Source: three-view drawing plus pictorial views. Frame: mm from the lowest corner of the part. A direction names the side the tool comes from. Round coordinates to 2 decimals unless told otherwise and drop trailing zeros. Order: outer loops, then holes, each group sorted by start corner. A loop starts at its lowest first (then second) coordinate and runs counter-clockwise, first axis right, second up. Notation, with made-up numbers: (4.25, -32) -> (58.25, -32) arc R24 cw to (58.25, 7) -> close; hole circle Ø9 at (-14, -23.5). An arc over 180 degrees is marked (long way). Use a Markdown table: item, result.
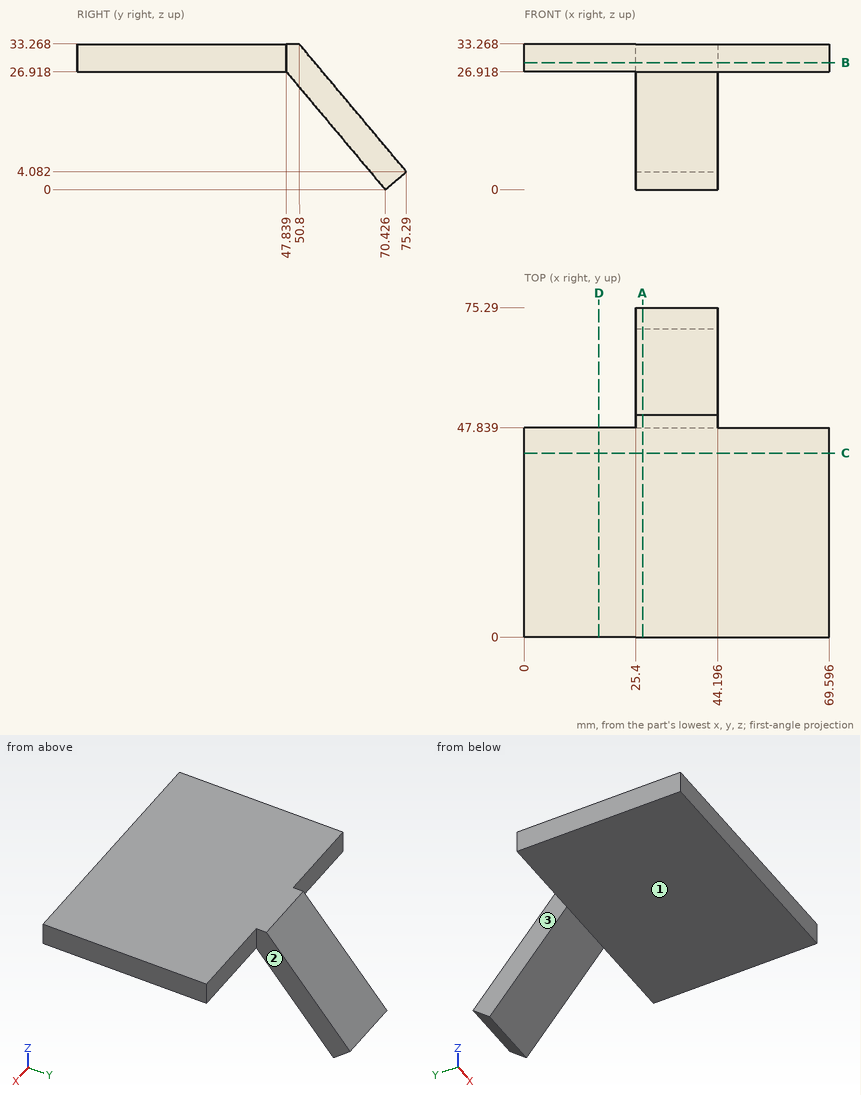
1) Line query: L1, parallel to X at y = 61.5, z = 17; L2, parallel to Z at x = 35, y = 35; L3, parallel to Y at x = 64.5, z = 27.5. Output: solid intervals per line, ascending. Write a range as [from, to].
Results found:
| item | result |
|---|---|
| L1 | x = [25.4, 44.2] |
| L2 | z = [26.92, 33.27] |
| L3 | y = [0, 47.84] |
2) Cut plane C-C on y = 42. Return loops of the section in (x, z).
Results found:
| item | result |
|---|---|
| outline | (0, 26.92) -> (69.6, 26.92) -> (69.6, 33.27) -> (0, 33.27) -> close |
3) Cut plane D-D on x = 17. Return loops of the section in (y, z), and give its area (3 significant figures).
Results found:
| item | result |
|---|---|
| outline | (0, 26.92) -> (47.84, 26.92) -> (47.84, 33.27) -> (0, 33.27) -> close |
| area | 304 mm² |
4) Set-up query: the marked faces 1, 2 and 3. Return all of +Z, -Z, +X, -X, +Y, -Y with unobstructed straight access to the full face (end or side cutting, diameter ignored); none if empty.
Results found:
| item | result |
|---|---|
| face 1 | -Z, +X, -X, -Y |
| face 2 | +Z, -Z, +X, +Y |
| face 3 | +Z, -Z, -X, +Y |
5) Pin query (flat end, axial travel): pin 1 Ø5 at (x, z) = (11.5, 31.5) entering from +Y; pin 2 Ø5 at (x, y) = (62, 49.5) entering from -Z; pin 3 Ø13.5 at (y, z) = (59, 9.5) entering from +X. Return the tip coordinate at first contact, or that it passes through.
Results found:
| item | result |
|---|---|
| pin 1 | stops at y = 47.84 |
| pin 2 | stops at z = 26.92 |
| pin 3 | stops at x = 44.2 |
6) Cut plane B-B on z = 29. Return loops of the section in (x, y), and give its area (3 significant figures).
Results found:
| item | result |
|---|---|
| outline | (0, 0) -> (69.6, 0) -> (69.6, 47.84) -> (44.2, 47.84) -> (44.2, 54.38) -> (25.4, 54.38) -> (25.4, 47.84) -> (0, 47.84) -> close |
| area | 3,450 mm² |
7) Cut plane A-A on x = 27. Return loops of the section in (y, z), and give its area (3 significant figures).
Results found:
| item | result |
|---|---|
| outline | (0, 26.92) -> (47.84, 26.92) -> (70.43, 0) -> (75.29, 4.08) -> (50.8, 33.27) -> (0, 33.27) -> close |
| area | 546 mm² |
